```python
from build123d import *

# Parameters (mm, degrees)
SKETCH8_R           = 2.5
BOSS_EXTRUDE4_DEPTH = 10


with BuildPart() as part:
    # Sketch8 → Boss-Extrude4 (new body)
    with BuildSketch(Plane.XY):
        with BuildLine():
            Line((9.877608164, 0), (9.877608164, 10))
            Line((9.877608164, 10), (-11.482689494, 10))
            Line((-11.482689494, 10), (-9.108332934, 16.523491033))
            Line((-9.108332934, 16.523491033), (-18.505259142, 19.943692467))
            Line((-18.505259142, 19.943692467), (-38.139157526, -34))
            add(Edge.make_bspline(
                [(-38.139157526, -34), (-28.952640902, -33.410718861), (-25.255337047, -27.84003816)],
                knots=[0, 0, 0, 0.686191173, 0.686191173, 0.686191173], degree=2))
            Line((-25.255337047, -27.84003816), (-15.122391836, 0))
            Line((-15.122391836, 0), (9.877608164, 0))
        make_face()
        with Locations((-15.711667653, 13)):
            Circle(SKETCH8_R, mode=Mode.SUBTRACT)
    extrude(amount=BOSS_EXTRUDE4_DEPTH)


solid = part.part
```
Input: part model. Units: mm. Frame: model coordinates. A direction names the side the tool comes from. Round coordinates to 2 decimals unless told otherwise and drop trailing zeros. Loops run counter-clockwise (first coordinate to the right, second up) from the corner with the lowest first, then second, coordinate; pieces in that order, holes last.
1) Section query C-C on y = 6.5. Return the cut outline in (x, z).
Ans:
outline: (-23.4, 0) - (9.88, 0) - (9.88, 10) - (-23.4, 10) - close
2) Set-up query: faces 4 (the flat face through (-10.31, 13.22, 4.93)), 5 (the flat face through (9.878, 5, 5)), 6 (the flat face through (-3, 0, 5)). Return all of +Z, -Z, +X, -X, +Y, -Y with unobstructed straight access to the full face (end or side cutting, diameter ignored); none if empty.
Ans:
face 4: +Z, -Z, +X
face 5: +Z, -Z, +X, +Y, -Y
face 6: +Z, -Z, +X, -Y
3) Section query A-A on y = 13. Return the cut outline in (x, z), plus the area to 3 significant figures.
Ans:
outline: (-21.03, 0) - (-18.21, 0) - (-18.21, 10) - (-21.03, 10) - close; (-13.21, 0) - (-10.39, 0) - (-10.39, 10) - (-13.21, 10) - close
area: 56.4 mm2
4) Pin query (flat end, axial travel): pin 1 (5 mm diameter, centred on y = -20, z = 1.5, fed in from -X); pin 2 (1 mm diameter, centred on x = 3, z = 4.5, fed in from -Y); pin 3 (5 mm diameter, centred on y = -7.5, z = 5.5, fed in from -X); pin 4 (4 mm diameter, centred on x = -15.71, y = 13, fed in from +Z). Return the tip coordinate at first contact, or that it passes through.
Ans:
pin 1: stops at x = -33.95
pin 2: stops at y = 0
pin 3: stops at x = -29.4
pin 4: passes through
5) Section query B-B on x = -5. Return the cut outline in (y, z).
Ans:
outline: (0, 0) - (10, 0) - (10, 10) - (0, 10) - close
6) Material intervals for line 1 (Y direction, x = -8, z = 4.5); line 2 (X direction, y = -13.5, z = 2.75); line 3 (X direction, y = -16.5, z = 4.5), sorted ascending.
Ans:
line 1: y = 0 to 10
line 2: x = -30.68 to -20.04
line 3: x = -31.77 to -21.13
7) Pull-direction query (Y, two-part tool) for faces 1 (the flat face through (-18, -5, 0)), 2 (the flat face through (-13.74, 18.21, 4.93)), 3 (the cylindrical face through (-16.25, 10.56, 4.93)); classes: released by +Y, released by -Y, zero draft, split by the parting line, or undercut.
Ans:
face 1: zero draft
face 2: released by +Y
face 3: undercut
